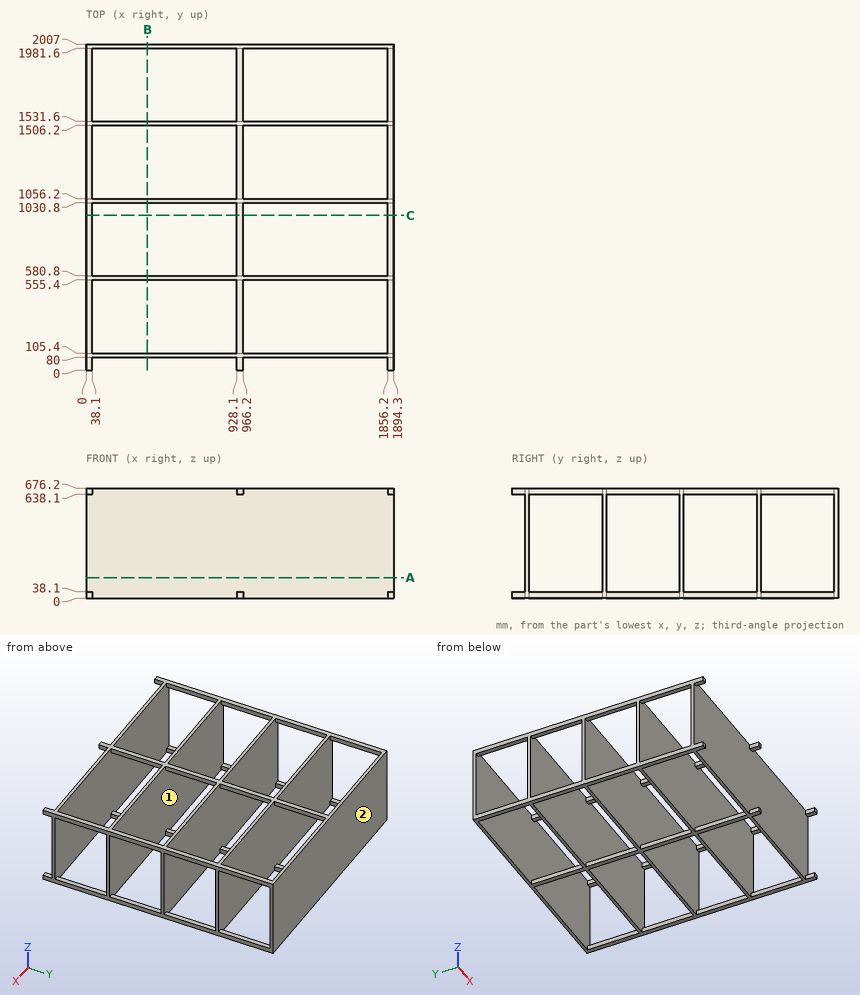
Study the drawing (mm; zero at the part's minimum x, y, z) and answer. Give positions to 0.01 mm unless a question says otherwise; leave off trailing zeros. Write each loop counter-clockwise with the first axis right and the second up, starting at its lowest first coordinate (ties: lowest second). Pieces come first, ordered by that corner, then holes. Notation, with made-up numbers: (-21.75, 53) - (37.25, 53) arc R14 cw to (37.25, 65) - close; hole circle Ø4 at (-21, 12). An arc over 180 degrees is marked (long way). One line per question, with ' | ' between items. Start each with the question number.
1. Given P1, Ø5, axis at x = 793.5, z = 499.5, coming from the -Y side, flat-ended and moving along its own axis, determine where the tip first touches the part or whether it passes through.
2. Section A-A, the plane z = 125 is taken. Determine the outline of the cut face in (x, y).
3. Determine the mould class of the marked faces 1 and 2 for opening direction Y: +Y half, -Y half, draft (parallel to the pull), parting line (faces both ways), or undercut.
4. Section C-C, the plane y = 953 is taken. Determine the outline of the cut face in (x, z).
5. Section B-B, the plane x = 377 is taken. Determine the outline of the cut face in (y, z), then the cut area to 3 significant figures.
6. Straight lines are drawn through the part: line 1 (Y direction, x = 1079.5, z = 450); line 2 (Z direction, x = 945, y = 257.5). For each, find the intervals that lie inside material, in ascending order.
Result:
1) P1: stops at y = 80
2) outline: (0, 80) - (1894.3, 80) - (1894.3, 105.4) - (0, 105.4) - close; (0, 555.4) - (1894.3, 555.4) - (1894.3, 580.8) - (0, 580.8) - close; (0, 1030.8) - (1894.3, 1030.8) - (1894.3, 1056.2) - (0, 1056.2) - close; (0, 1506.2) - (1894.3, 1506.2) - (1894.3, 1531.6) - (0, 1531.6) - close; (0, 1981.6) - (1894.3, 1981.6) - (1894.3, 2007) - (0, 2007) - close
3) face 1: undercut | face 2: +Y half
4) outline: (0, 0) - (38.1, 0) - (38.1, 38.1) - (0, 38.1) - close; (0, 638.1) - (38.1, 638.1) - (38.1, 676.2) - (0, 676.2) - close; (928.1, 0) - (966.2, 0) - (966.2, 38.1) - (928.1, 38.1) - close; (928.1, 638.1) - (966.2, 638.1) - (966.2, 676.2) - (928.1, 676.2) - close; (1856.2, 0) - (1894.3, 0) - (1894.3, 38.1) - (1856.2, 38.1) - close; (1856.2, 638.1) - (1894.3, 638.1) - (1894.3, 676.2) - (1856.2, 676.2) - close
5) outline: (80, 0) - (105.4, 0) - (105.4, 676.2) - (80, 676.2) - close; (555.4, 0) - (580.8, 0) - (580.8, 676.2) - (555.4, 676.2) - close; (1030.8, 0) - (1056.2, 0) - (1056.2, 676.2) - (1030.8, 676.2) - close; (1506.2, 0) - (1531.6, 0) - (1531.6, 676.2) - (1506.2, 676.2) - close; (1981.6, 0) - (2007, 0) - (2007, 676.2) - (1981.6, 676.2) - close | area: 85,900 mm2
6) line 1: y = 80 to 105.4, 555.4 to 580.8, 1030.8 to 1056.2, 1506.2 to 1531.6, 1981.6 to 2007 | line 2: z = 0 to 38.1, 638.1 to 676.2
